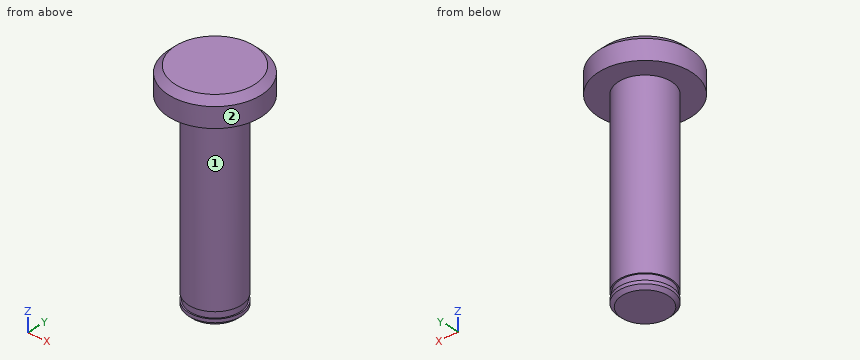
```python
from build123d import *


with BuildPart() as part:
    # Esquisse3 → Base-Révolution (revolve)
    with BuildSketch(Plane(origin=(0, 0, 0), x_dir=(1, 0, 0), z_dir=(0, 1, 0)), mode=Mode.PRIVATE) as base_r_volution_sk:
        Polygon((-14.488580903, -38.951150448), (-8.488580903, -38.951150448), (-8.488580903, -5.951150448), (-11.988580903, -5.951150448), (-12.488580903, -6.451150448), (-12.488580903, -6.951150448), (-12.288580903, -6.951150448), (-12.288580903, -7.951150448), (-12.488580903, -7.951150448), (-12.488580903, -34.951150448), (-15.488580903, -34.951150448), (-15.488580903, -37.951150448), align=None)
    revolve(base_r_volution_sk.sketch.rotate(Axis((-8.488580903, 0, 56.293331626), (0, 0, -1)), 180), axis=Axis((-8.488580903, 0, 56.293331626), (0, 0, -1)))


solid = part.part
```
Source: CAD feature listing. Evaluate the final solid. Frame: model axes, mm. Face numbers are marked on the shaded views. A direction names the side the tool comes from. Coordinates: 2 decimals unless noted, no trailing zeros. Loops run counter-clockwise (first coordinate to the right, second up) from the corner with the lowest first, then second, coordinate; pieces in that order, holes last. Notation, with made-up numbers: M -20,74.25 L 33,74.25 A11 cw 33,86.25 Z; hole C 81.25,-14 d1. An arc over 180 degrees is marked long. Put each result on its own line as item: value. Start each with the question number.
1) Contact query for flat-ended pins moving along their axis: pin 1 Ø2 at (y, z) = (-2, 26.5) entering from -X; pin 2 Ø1.5 at (x, z) = (-4, 34.5) entering from +Y; pin 3 Ø1.5 at (x, z) = (-10.5, 33) entering from +Y. Output: stop coordinate, or through.
2) Cut plane B-B on z = 22. Return the cut outline in (x, y).
3) Cut plane A-A on y = 0. Return the cut outline in (x, z), then the cut area to 3 significant figures.
4) Ray query, L1, parallel to X at y = 1.25, z = 11; L2, parallel to Z at x = -5.25, y = 4.25; L3, parallel to X at y = -1.75, z = 28.5. Return the intervals inside material, ascending. Write a range as from..to.
5) Reachability of the marked faces 1 and 2 from +Z, -Z, +X, -X, +Y, -Y: full face, straight path, thin tool, end or side. Return the list, or none.
The answers:
1. pin 1: stops at x = -12.36
1. pin 2: stops at y = 5.82
1. pin 3: stops at y = 3.8
2. outline: C -8.49,0 d8
3. outline: M -15.49,34.95 L -12.49,34.95 L -12.49,7.95 L -12.29,7.95 L -12.29,6.95 L -12.49,6.95 L -12.49,6.45 L -11.99,5.95 L -4.99,5.95 L -4.49,6.45 L -4.49,6.95 L -4.69,6.95 L -4.69,7.95 L -4.49,7.95 L -4.49,34.95 L -1.49,34.95 L -1.49,37.95 L -2.49,38.95 L -14.49,38.95 L -15.49,37.95 Z
3. area: 286 mm²
4. L1: x = -12.29..-4.69
4. L2: z = 34.95..38.95
4. L3: x = -12.09..-4.89
5. face 1: -Z
5. face 2: +Z, -Z
